Source: CAD feature listing. Evaluate the final solid. Frame: model axes, mm. A direction names the side the tool comes from. Round coordinates to 2 decimals unless told otherwise and drop trailing zeros. Order: outer loops, then holes, each group sorted by start corner. A loop starts at its lowest first (then second) coordinate and runs counter-clockwise, first axis right, second up. Notation, with made-up numbers: M 37,26 L 92,26 A17 ccw 92,40 Z; hole C 48,17.5 d6. An arc over 180 degrees is marked long. Answer as CSV lines item,"result". Start each with the question number.
Item 1: Section query C-C on x = 0. Return the cut outline in (y, z) (3 decimals), plus the area to 3 significant figures.
Item 2: Line query: line 1 (X direction, y = 23.25, z = 0) (3 decimals); line 2 (Y direction, x = -5.25, z = 1.75); line 3 (X direction, y = 15.5, z = -8.25). Output: solid intervals per line, ascending. Write a range as [from, to].
Item 3: Section query B-B on y = 26.5. Return the cut outline in (x, z) (3 decimals).
Item 4: Pull-direction query (Z, two-part tool) for faces 3 (the face through (0, 0, 8)), 4 (the face through (-0.17, 29.9, -1.26)), 5 (the face through (-0.31, 14.613, -10.282)); classes: +Z half, -Z half, draft (parallel to the pull), parting line (faces both ways), or undercut.
Item 5: Section query D-D on z = -7. Return the cut outline in (x, y), plus the area to 3 significant figures.
Item 6: First-contact query: P1, Ø5, axis at y = 17, z = -8, coming from the -X side; P2, Ø1.5, axis at y = 26, z = -8, coming from the -X side; P3, Ø1.5, axis at x = -4.5, y = 20, coming from the -Z side. Flat tips, straight axial feed; report the tip coordinate or a pass-through.
Item 7: Set-up query: faces 1 (the face through (0, 29.642, 2)), 2 (the face through (0, 30.15, 2)). Return all of +Z, -Z, +X, -X, +Y, -Y with unobstructed straight access to the full face (end or side cutting, diameter ignored); none if empty.
Item 8: Section query A-A on x = 6.25. Return the cut outline in (y, z), plus the area to 3 significant figures.
from build123d import *

# Parameters (mm, degrees)
SKETCH1_R           = 10.795
SKETCH1_R_2         = 10.287
BOSS_EXTRUDE1_DEPTH = 29.6418
BOSS_EXTRUDE3_DEPTH = 0.508
SKETCH3_R           = 1.27
CUT_EXTRUDE1_DEPTH  = 31.1498
BOSS_EXTRUDE4_REACH = 32.15


with BuildPart() as part:
    # Sketch1 → Boss-Extrude1 (new body)
    with BuildSketch(Plane(origin=(0, 0, 0), x_dir=(1, 0, 0), z_dir=(0, 1, 0))):
        Circle(SKETCH1_R)
        Circle(SKETCH1_R_2, mode=Mode.SUBTRACT)
    extrude(amount=BOSS_EXTRUDE1_DEPTH)

    # Sketch2 → Boss-Extrude3 (add)
    with BuildSketch(Plane(origin=(0, 29.6418, 0), x_dir=(1, 0, 0), z_dir=(0, 1, 0))):
        with BuildLine():
            Line((8.451883262, 5.864131507), (-9.126833577, 4.745869558))
            ThreePointArc((-9.126833577, 4.745869558), (-2.442809038, -9.992750022), (10.287, 0))
            ThreePointArc((10.287, 0), (9.81750712, 3.072283018), (8.451883262, 5.864131507))
        make_face()
        with BuildLine():
            Line((-9.126833577, 4.745869558), (-9.714005015, 4.708516918))
            ThreePointArc((-9.714005015, 4.708516918), (-2.415506247, -10.521281033), (10.795, 0))
            ThreePointArc((10.795, 0), (10.346705284, 3.078589735), (9.0390547, 5.901484146))
            Line((9.0390547, 5.901484146), (8.451883262, 5.864131507))
            ThreePointArc((8.451883262, 5.864131507), (9.81750712, 3.072283018), (10.287, 0))
            ThreePointArc((10.287, 0), (-2.442809038, -9.992750022), (-9.126833577, 4.745869558))
        make_face()
    extrude(amount=BOSS_EXTRUDE3_DEPTH)

    # Sketch3 → Cut-Extrude1 (cut, through all)
    with BuildSketch(Plane(origin=(0, 30.1498, 0), x_dir=(1, 0, 0), z_dir=(0, 1, 0))):
        Circle(SKETCH3_R)
    extrude(amount=-CUT_EXTRUDE1_DEPTH, mode=Mode.SUBTRACT)

    # Sketch6 → Boss-Extrude4 (add, up to next)
    with BuildSketch(Plane.XZ, mode=Mode.PRIVATE) as boss_extrude4_sk1:
        with BuildLine():
            Line((-3.869377765, 7.761308892), (4.821670905, 7.208431847))
            Line((4.821670905, 7.208431847), (7.502708149, 7.037878901))
            ThreePointArc((7.502708149, 7.037878901), (0.653082635, 10.266248198), (-6.550415009, 7.931861837))
            Line((-6.550415009, 7.931861837), (-3.869377765, 7.761308892))
        make_face()
    boss_extrude4_tool1 = extrude(boss_extrude4_sk1.sketch, amount=-BOSS_EXTRUDE4_REACH, mode=Mode.PRIVATE) - part.part
    add(boss_extrude4_tool1.solids().sort_by_distance((0.547813, 0, 8.611444))[0])


solid = part.part
Results:
1,outline,"M 0,-10.795 L 29.642,-10.795 L 29.642,-10.287 L 0,-10.287 Z; M 0,7.515 L 29.642,7.515 L 29.642,1.27 L 30.15,1.27 L 30.15,10.795 L 0,10.795 Z; M 29.642,-5.326 L 30.15,-5.326 L 30.15,-1.27 L 29.642,-1.27 Z"
1,area,"119 mm^2"
2,line 1,"[-10.795, -10.287], [10.287, 10.795]"
2,line 2,"[29.64, 30.15]"
2,line 3,"[-6.96, -6.14], [6.14, 6.96]"
3,outline,"C 0,0 d21.59; hole M -6.55,7.932 A10.287 ccw long 7.503,7.038 Z"
4,face 3,"draft"
4,face 4,"undercut"
4,face 5,"undercut"
5,outline,"M -8.22,0 L -7.54,0 L -7.54,29.64 L -8.22,29.64 Z; M 7.54,0 L 8.22,0 L 8.22,29.64 L 7.54,29.64 Z"
5,area,"40.3 mm^2"
6,P1,"x = -9.29"
6,P2,"x = -8"
6,P3,"z = -10.12"
7,face 1,"-Y"
7,face 2,"+Z, -Z, +X, -X, +Y"
8,outline,"M 0,-8.8 L 29.64,-8.8 L 29.64,-8.17 L 0,-8.17 Z; M 0,7.12 L 29.64,7.12 L 29.64,-5.72 L 30.15,-5.72 L 30.15,8.8 L 0,8.8 Z"
8,area,"76.0 mm^2"
